from build123d import *

# Parameters (mm, degrees)
SKETCH1_W                             = 37
SKETCH1_H                             = 63
BOSS_EXTRUDE1_DEPTH                   = 8
SKETCH2_R                             = 1
CUT_EXTRUDE1_DEPTH                    = 10
SKETCH3_W                             = 10
SKETCH3_H                             = 8
BOSS_EXTRUDE2_DEPTH                   = 37
CUT_EXTRUDE2_REACH                    = 68.417
SKETCH4_W                             = 26.5
SKETCH4_H                             = 50
M3_CLEARANCE_HOLE1_AT_2_COUNT         = 2
M3_CLEARANCE_HOLE1_AT_2_PITCH         = 29
M3_CLEARANCE_HOLE1_AT_3_COUNT         = 2
M3_CLEARANCE_HOLE1_AT_3_PITCH         = 17.613914954
FILLET1_R                             = 2
SKETCH8_W                             = 25
SKETCH8_H                             = 8
BOSS_EXTRUDE3_DEPTH                   = 8
SKETCH9_R                             = 1
CUT_EXTRUDE3_DEPTH                    = 5
TAP_DRILL_FOR_M3X0_5_TAP1_D           = 2.5
TAP_DRILL_FOR_M3X0_5_TAP1_CSINK_D     = 2.55
TAP_DRILL_FOR_M3X0_5_TAP1_CSINK_ANGLE = 90
M3_CLEARANCE_HOLE2_D                  = 3.6
M3_CLEARANCE_HOLE2_CSINK_D            = 3.65
M3_CLEARANCE_HOLE2_CSINK_ANGLE        = 90


with BuildPart() as part:
    # Sketch1 → Boss-Extrude1 (new body)
    with BuildSketch(Plane.XY):
        with Locations((0, 31.5)):
            Rectangle(SKETCH1_W, SKETCH1_H)
    extrude(amount=BOSS_EXTRUDE1_DEPTH)

    # Sketch2 → Cut-Extrude1 (cut)
    with BuildSketch(Plane.ZY.offset(18.5)):
        with Locations((4, 51.5)):
            Circle(SKETCH2_R)
        with Locations((4, 11.5)):
            Circle(SKETCH2_R)
    cut_extrude1 = extrude(amount=-CUT_EXTRUDE1_DEPTH, mode=Mode.SUBTRACT)

    # Mirror1: Cut-Extrude1 across plane
    add(cut_extrude1.mirror(Plane(origin=(0, 0, 0), x_dir=(0, 0, 1), z_dir=(1, 0, 0))), mode=Mode.SUBTRACT)

    # Sketch3 → Boss-Extrude2 (add)
    with BuildSketch(Plane.ZY.offset(18.5)):
        with Locations((13, 4)):
            Rectangle(SKETCH3_W, SKETCH3_H)
    extrude(amount=-BOSS_EXTRUDE2_DEPTH)

    # Sketch4 → Cut-Extrude2 (cut, up to next)
    with BuildSketch(Plane.XY.offset(8), mode=Mode.PRIVATE) as cut_extrude2_sk1:
        with Locations((0, 33)):
            Rectangle(SKETCH4_W, SKETCH4_H)
    cut_extrude2_tool1 = extrude(cut_extrude2_sk1.sketch, amount=-CUT_EXTRUDE2_REACH, mode=Mode.PRIVATE) & part.part
    add(cut_extrude2_tool1.solids().sort_by_distance((0, 33, 8))[0], mode=Mode.SUBTRACT)

    # Sketch7 → M3 Clearance Hole1 (revolve, cut)
    with BuildSketch(Plane(origin=(-14.5, 8, 14), x_dir=(0, 0, 1), z_dir=(1, 0, 0))):
        Polygon((0, 0), (0, 8), (1.725, 8), (1.7, 7.975), (1.7, 0.025), (1.725, 0), align=None)
    m3_clearance_hole1 = revolve(axis=Axis((-14.5, 14.35, 14), (0, -1, 0)), mode=Mode.SUBTRACT)

    # M3 Clearance Hole1 at 2: M3 Clearance Hole1 ×2
    with Locations(*[(i * M3_CLEARANCE_HOLE1_AT_2_PITCH, 0, 0) for i in range(1, M3_CLEARANCE_HOLE1_AT_2_COUNT)]):
        add(m3_clearance_hole1, mode=Mode.SUBTRACT)

    # M3 Clearance Hole1 at 3: M3 Clearance Hole1 ×2
    with Locations(*[Vector(0.8232127859153063, 0, -0.5677329558036597) * (i * M3_CLEARANCE_HOLE1_AT_3_PITCH) for i in range(1, M3_CLEARANCE_HOLE1_AT_3_COUNT)]):
        add(m3_clearance_hole1, mode=Mode.SUBTRACT)

    # Fillet1
    fillet1_edges = [part.edges().sort_by_distance(p)[0] for p in [
        (15.875, 8, 8),
        (-15.875, 8, 8),
        (-13.25, 8, 4),
        (-13.25, 58, 4),
        (13.25, 58, 4),
        (13.25, 8, 4),
    ]]
    fillet(fillet1_edges, radius=FILLET1_R)

    # Sketch8 → Boss-Extrude3 (add)
    with BuildSketch(Plane(origin=(0, 0, 0), x_dir=(-1, 0, 0), z_dir=(0, 0, -1))):
        with Locations((0, 67)):
            Rectangle(SKETCH8_W, SKETCH8_H)
    extrude(amount=-BOSS_EXTRUDE3_DEPTH)

    # Sketch9 → Cut-Extrude3 (cut)
    with BuildSketch(Plane.ZY.offset(12.5)):
        with Locations(Location((4, 67, 0), (0, 0, 270))):
            Circle(SKETCH9_R)
    cut_extrude3 = extrude(amount=-CUT_EXTRUDE3_DEPTH, mode=Mode.SUBTRACT)

    # Mirror2: Cut-Extrude3 across plane
    add(cut_extrude3.mirror(Plane(origin=(0, 0, 0), x_dir=(0, 0, 1), z_dir=(1, 0, 0))), mode=Mode.SUBTRACT)

    # Tap Drill for M3x0.5 Tap1 (through all)
    with Locations(Plane.ZY.offset(18.5)):
        with Locations((4, 11.5)):
            CounterSinkHole(TAP_DRILL_FOR_M3X0_5_TAP1_D / 2, TAP_DRILL_FOR_M3X0_5_TAP1_CSINK_D / 2, counter_sink_angle=TAP_DRILL_FOR_M3X0_5_TAP1_CSINK_ANGLE)

    # M3 Clearance Hole2 (through all)
    with Locations(Plane.ZY.offset(18.5)):
        with Locations((4, 51.5)):
            CounterSinkHole(M3_CLEARANCE_HOLE2_D / 2, M3_CLEARANCE_HOLE2_CSINK_D / 2, counter_sink_angle=M3_CLEARANCE_HOLE2_CSINK_ANGLE)

    # Sketch15 → Tap Drill for M3x0.5 Tap2 (revolve, cut)
    with BuildSketch(Plane(origin=(-12.5, 67, 4), x_dir=(0, 0, 1), z_dir=(0, 1, 0))):
        Polygon((0, 0), (0, 20.751075774), (1.25, 20), (1.25, 0.025), (1.275, 0), align=None)
    tap_drill_for_m3x0_5_tap2 = revolve(axis=Axis((-18.85, 67, 4), (1, 0, 0)), mode=Mode.SUBTRACT)

    # Mirror3: Tap Drill for M3x0.5 Tap2 across plane
    add(tap_drill_for_m3x0_5_tap2.mirror(Plane(origin=(0, 0, 0), x_dir=(0, 0, 1), z_dir=(1, 0, 0))), mode=Mode.SUBTRACT)


solid = part.part
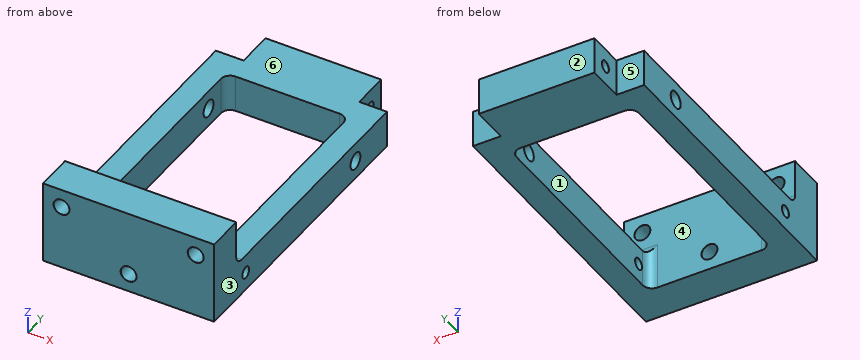
Could you check a few things on this model? Use its own coordinates, in mm. Face numbers are marked on the shaded views. A direction names the side the tool comes from. Coordinates: 2 decimals unless noted, no trailing zeros. Order: outer loops, then holes, each group sorted by start corner. A loop starts at its lowest first (then second) coordinate and runs counter-clockwise, first axis right, second up. Notation, with made-up numbers: (-11.5, 16.5) -> (7.5, 16.5) arc R23 cw to (7.5, 52.5) -> close; hole circle Ø9 at (66.5, -10.75). An arc over 180 degrees is marked (long way). One line per question, with ' | ' between items.
Q1. I'm going to push flat-ended pins straight in: P1, Ø4, axis at y = 67, z = 5.5, coming from the -X side; P2, Ø4, axis at y = 11.5, z = 4, coming from the -X side; P3, Ø1.8, axis at x = -16.5, z = 5.5, coming from the +Y side; P4, Ø1.5, axis at x = -13.5, y = 63.5, coming from the +Z side. Where does each tip first touch, or does it pass through?
Return value:
P1: x = -12.5 | P2: x = -18.5 | P3: y = 63 | P4: z = 8
Q2. Thinking about a two-plate mould opening in X: for the marked faces 1, 2 and 3, which applies, pulls with the +X half, pulls with the -X half, needs draft (parallel to the pull), parting line crosses it, or undercut?
Return value:
face 1: undercut | face 2: needs draft | face 3: pulls with the +X half
Q3. If I drill on L1, parallel to X at y = 4.25, z = 14; L2, parallel to Y at x = -17.2, z = 4; L3, parallel to Y at x = -7, z = 4, over which ranges is the centre line in solid material (lowest first)?
Return value:
L1: -18.5 to -16.2, -12.8 to 12.8, 16.2 to 18.5 | L2: 0 to 10.25, 12.75 to 49.7, 53.3 to 63 | L3: 0 to 8, 58 to 65.75, 68.25 to 71
Q4. Imagine slicing it at C-C on x = 0. Please give me the cut outline in (y, z) (3 decimals), and give its area (3 significant figures).
Return value:
outline: (0, 0) -> (8, 0) -> (8, 2.275) -> (7.975, 2.3) -> (0.025, 2.3) -> (0, 2.275) -> close; (0, 5.725) -> (0.025, 5.7) -> (7.975, 5.7) -> (8, 5.725) -> (8, 18) -> (0, 18) -> close; (58, 0) -> (71, 0) -> (71, 8) -> (58, 8) -> close; hole circle Ø2.5 at (67, 4) | area: 216 mm²
Q5. On a 3-axis mill with a long thin cutter (end or side, diameter ignored), from which of +Z, -Z, +X, -X, +Y, -Y can I reach the whole of each face in a straight line? I mean the marked faces 4, 5 and 6. Say none if no direction works.
Return value:
face 4: +Z | face 5: +Z, -Z, -X, +Y | face 6: +Z, +X, -X, +Y
Q6. Imagine slicing it at A-A on x = 8. Please give me the cut outline in (y, z), and give its area (3 significant figures).
Return value:
outline: (0, 0) -> (8, 0) -> (8, 18) -> (0, 18) -> close; (58, 0) -> (71, 0) -> (71, 8) -> (58, 8) -> close; hole circle Ø2.5 at (67, 4) | area: 243 mm²
Q7. Imagine slicing it at D-D on x = 14.5. Please give me the cut outline in (y, z) (3 decimals), and give its area (3 significant figures).
Return value:
outline: (0, 0) -> (63, 0) -> (63, 8) -> (10, 8) arc R2 cw to (8, 10) -> (8, 12.275) -> (7.975, 12.3) -> (0.025, 12.3) -> (0, 12.275) -> close; (0, 15.725) -> (0.025, 15.7) -> (7.975, 15.7) -> (8, 15.725) -> (8, 18) -> (0, 18) -> close; hole circle Ø2.5 at (11.5, 4); hole circle Ø3.6 at (51.5, 4) | area: 543 mm²
Q8. Imagine slicing it at B-B on y = 11.5. Please give me the cut outline in (x, z) (3 decimals).
Return value:
outline: (-18.5, 0) -> (-13.25, 0) -> (-13.25, 2.75) -> (-18.475, 2.75) -> (-18.5, 2.725) -> close; (-18.5, 5.275) -> (-18.475, 5.25) -> (-13.25, 5.25) -> (-13.25, 8) -> (-18.5, 8) -> close; (13.25, 0) -> (18.5, 0) -> (18.5, 2.75) -> (13.25, 2.75) -> close; (13.25, 5.25) -> (18.5, 5.25) -> (18.5, 8) -> (13.25, 8) -> close
